from build123d import *

# Parameters (mm, degrees)
F0_W     = 22.098
F0_H     = 4.318
F0_W_2   = 2.032
F0_H_2   = 1.27
F0_W_3   = 1.016
F1_DEPTH = 12.7
F2_DEPTH = 12.7


# Not quite as in the source:
# - a feature names something its author has since deleted; it is built from what else it names


with BuildPart() as f1:
    # F0 (on Top) → F1 (new body)
    with BuildSketch(Plane.XY):
        with Locations((-31.8938936177, -48.641)):
            Rectangle(F0_W, F0_H)
        with Locations((-43.9588936177, -48.641)):
            Rectangle(F0_W_2, F0_H)
        with Locations((-31.8938936177, -51.435)):
            Rectangle(F0_W, F0_H_2)
        with Locations((-31.8938936177, -45.847)):
            Rectangle(F0_W, F0_H_2)
        with Locations((-20.3368936177, -48.641)):
            Rectangle(F0_W_3, F0_H)
        Polygon((-50.8410629748, -50.8), (-44.9748936177, -50.8), (-44.9748936177, -46.482), (-44.9748936177, 34.798), (-44.9748936177, 39.116), (-50.8410629748, 39.116), align=None)
    extrude(amount=F1_DEPTH)

    # F0 (on Top) → F2 (join)
    with BuildSketch(Plane.XY):
        with Locations((-31.8938936177, 36.957)):
            Rectangle(F0_W, F0_H)
        with Locations((-43.9588936177, 36.957)):
            Rectangle(F0_W_2, F0_H)
        with Locations((-31.8938936177, 34.163)):
            Rectangle(F0_W, F0_H_2)
        with Locations((-31.8938936177, 39.751)):
            Rectangle(F0_W, F0_H_2)
        with Locations((-20.3368936177, 36.957)):
            Rectangle(F0_W_3, F0_H)
    extrude(amount=F2_DEPTH)


solid = f1.part
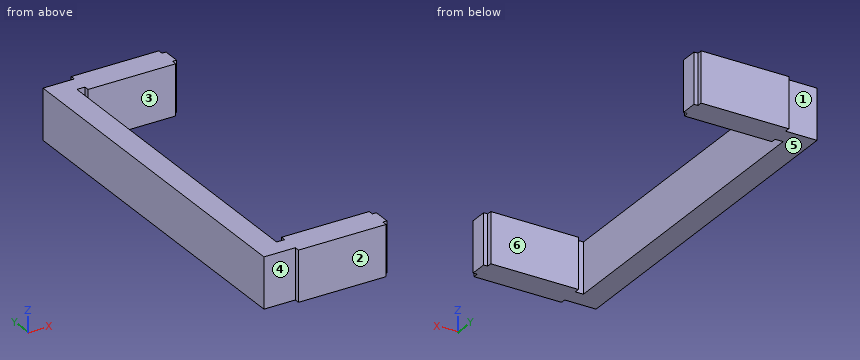
Check sheet for the modelled part. Datum: model origin and axes. Units: mm. Face numbers are marked on the shaded views. A direction names the side the tool comes from. Round coordinates to 2 decimals unless told otherwise and drop trailing zeros. Loops run counter-clockwise (first coordinate to the right, second up) from the corner with the lowest first, then second, coordinate; pieces in that order, holes last.
1. Gauge pin test, flat ends, axial feed: pin 1 Ø0.6 at (y, z) = (-51.5, 5) entering from +X; pin 2 Ø0.5 at (x, z) = (-20.5, 8.5) entering from +Y; pin 3 Ø0.6 at (y, z) = (40, 3.5) entering from -X. Record the tip position at first contact, or that the pin passes through.
2. Sectioned sample at C-C on x = -35.5. Record the boundary of the cut face in (y, z).
3. Sectioned sample at B-B on z = 5.5. Record the boundary of the cut face in (x, y).
4. Sectioned sample at D-D on y = -31. Record the boundary of the cut face in (x, z), and give its area (3 significant figures).
5. Sectioned sample at A-A on x = -44. Record the boundary of the cut face in (y, z), and give its area (3 significant figures).
6. Scan lines: probe 1 along Y at (x, z) = (-24, 8); probe 2 along X at (y, z) = (-44, 6.75); probe 3 along Y at (x, z) = (-49, 11.25). Record each from-to range of solid material in increasing order.
7. Mould release check, pull along Y, two halves, no side actions. Record for the marked faces 1, 2 and 3: released by +Y, released by -Y, zero draft, split by the parting line, or undercut.
8. Set-up check for the marked faces 4, 5 and 6: record each of +Z, -Z, +X, -X, +Y, -Y from which the full face is reachable in a straight line by a thin tool's end or side.
Recorded:
1. pin 1: stops at x = -20.84
1. pin 2: stops at y = 39.12
1. pin 3: stops at x = -42.94
2. outline: (-52.07, 0) - (-45.21, 0) - (-45.21, 12.7) - (-52.07, 12.7) - close; (33.53, 0) - (40.39, 0) - (40.39, 12.7) - (33.53, 12.7) - close
3. outline: (-50.84, -50.8) - (-42.94, -50.8) - (-42.94, -52.07) - (-20.84, -52.07) - (-20.84, -50.8) - (-19.83, -50.8) - (-19.83, -46.48) - (-20.84, -46.48) - (-20.84, -45.21) - (-42.94, -45.21) - (-42.94, -46.48) - (-44.97, -46.48) - (-44.97, 34.8) - (-42.94, 34.8) - (-42.94, 33.53) - (-20.84, 33.53) - (-20.84, 34.8) - (-19.83, 34.8) - (-19.83, 39.12) - (-20.84, 39.12) - (-20.84, 40.39) - (-42.94, 40.39) - (-42.94, 39.12) - (-50.84, 39.12) - close
4. outline: (-50.84, 0) - (-44.97, 0) - (-44.97, 12.7) - (-50.84, 12.7) - close
4. area: 74.5 mm2
5. outline: (-50.8, 0) - (-46.48, 0) - (-46.48, 12.7) - (-50.8, 12.7) - close; (34.8, 0) - (39.12, 0) - (39.12, 12.7) - (34.8, 12.7) - close
5. area: 110 mm2
6. probe 1: y = -52.07 to -45.21, 33.53 to 40.39
6. probe 2: x = -50.84 to -44.97
6. probe 3: y = -50.8 to 39.12
7. face 1: released by +Y
7. face 2: released by -Y
7. face 3: undercut
8. face 4: +Z, -Z, -X, -Y
8. face 5: -Z, +X, -X, +Y, -Y
8. face 6: +Z, -Z, +X
